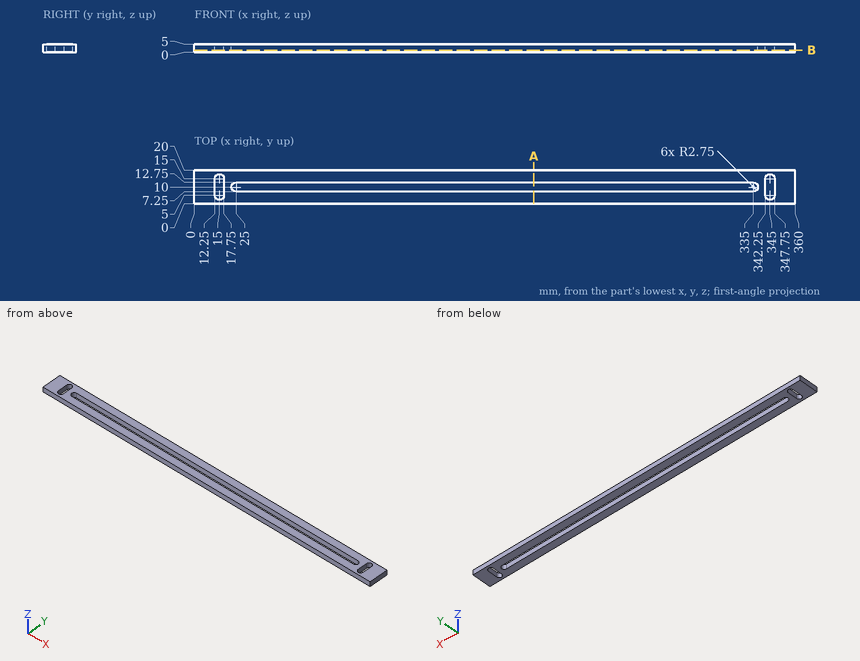
Design review of the part shown in the three views and the two pictorial views. Dimensions are in mm from the part's minimum x, y and z. Round coordinates to 2 decimals unless told otherwise and drop trailing zeros. Order: outer loops, then holes, each group sorted by start corner. A loop starts at its lowest first (then second) coordinate and runs counter-clockwise, first axis right, second up.
Item 1: Add section B-B, the plane z = 1.3. State the section outline as (x, y) points, and give its area (3 significant figures).
Working result:
outline: (0, 0) - (360, 0) - (360, 20) - (0, 20) - close; hole (12.25, 5) arc R2.75 ccw to (17.75, 5) - (17.75, 15) arc R2.75 ccw to (12.25, 15) - close; hole (25, 7.25) - (335, 7.25) arc R2.75 ccw to (335, 12.75) - (25, 12.75) arc R2.75 ccw to start; hole (342.25, 5) arc R2.75 ccw to (347.75, 5) - (347.75, 15) arc R2.75 ccw to (342.25, 15) - close
area: 5,310 mm2
Item 2: Add section A-A, the plane x = 203.5. State the section outline as (y, z) points.
Working result:
outline: (0, 0) - (7.25, 0) - (7.25, 5) - (0, 5) - close; (12.75, 0) - (20, 0) - (20, 5) - (12.75, 5) - close
Item 3: To check wall thickness, follow probe 1 along X at (y, z) = (6, 4.65); probe 2 along Y at (x, z) = (167, 2.6). State the ranges of each line that lie inside material, in increasing order.
Working result:
probe 1: x = 0 to 12.25, 17.75 to 342.25, 347.75 to 360
probe 2: y = 0 to 7.25, 12.75 to 20
Item 4: For pin 1 (1.5 mm diameter, centred on x = 216.5, y = 10.5, fed in from -Z), flat-tipped, find the tip position at first contact; note if it passes through.
Working result:
pin 1: passes through
